For this review, take the finished solid that the model builds, in its own axes (mm). A direction names the side the tool comes from. Round coordinates to 2 decimals unless told otherwise and drop trailing zeros. Write each loop counter-clockwise with the first axis right and the second up, starting at its lowest first coordinate (ties: lowest second). Pieces come first, ordered by that corner, then holes. Notation, with made-up numbers: M 37.25,13.5 L 74.25,13.5 A9 cw 74.25,29.5 Z; hole C 22,0.25 d11. An arc over 180 degrees is marked long. Answer in a Markdown table with one row per item.
```python
from build123d import *

# Parameters (mm, degrees)
SKETCH1_W                      = 170
SKETCH1_H                      = 200
BOSS_EXTRUDE1_DEPTH            = 3
FILLET1_R                      = 3
F_3_0MM_DOWEL_HOLE1_AT_2_COUNT = 2
F_3_0MM_DOWEL_HOLE1_AT_2_PITCH = 15
F_3_0MM_DOWEL_HOLE1_AT_3_COUNT = 2
F_3_0MM_DOWEL_HOLE1_AT_3_PITCH = 75
F_3_0MM_DOWEL_HOLE1_AT_4_COUNT = 2
F_3_0MM_DOWEL_HOLE1_AT_4_PITCH = 90
F_3_0MM_DOWEL_HOLE1_AT_5_COUNT = 2
F_3_0MM_DOWEL_HOLE1_AT_5_PITCH = 60
F_3_0MM_DOWEL_HOLE1_AT_6_COUNT = 2
F_3_0MM_DOWEL_HOLE1_AT_6_PITCH = 75
FILLET1_OF_MIRROR1_R           = 3


with BuildPart() as part:
    # Sketch1 → Boss-Extrude1 (new body)
    with BuildSketch(Plane(origin=(0, 0, 0), x_dir=(1, 0, 0), z_dir=(0, 1, 0))):
        with Locations((-85, 0)):
            Rectangle(SKETCH1_W, SKETCH1_H)
        Polygon((-19.723082923, 85.294117647), (-19.723082923, 23.203626969), (-125.276917077, 85.294117647), align=None, mode=Mode.SUBTRACT)
        Polygon((-39.446165847, 11.601813484), (-145, 11.601813484), (-145, 73.692304163), align=None, mode=Mode.SUBTRACT)
        Polygon((-125.276917077, -85.294117647), (-19.723082923, -23.203626969), (-19.723082923, -85.294117647), align=None, mode=Mode.SUBTRACT)
        Polygon((-145, -11.601813484), (-39.446165847, -11.601813484), (-145, -73.692304163), align=None, mode=Mode.SUBTRACT)
    boss_extrude1 = extrude(amount=BOSS_EXTRUDE1_DEPTH)

    # Fillet1
    fillet1_edges = [part.edges().sort_by_distance(p)[0] for p in [
        (-19.723082923, 1.5, -23.203626969),
        (-19.723082923, 1.5, -85.294117647),
        (-125.276917077, 1.5, -85.294117647),
        (-39.446165847, 1.5, -11.601813484),
        (-145, 1.5, -73.692304163),
        (-145, 1.5, -11.601813484),
        (-39.446165847, 1.5, 11.601813484),
        (-145, 1.5, 11.601813484),
        (-145, 1.5, 73.692304163),
        (-19.723082923, 1.5, 23.203626969),
        (-125.276917077, 1.5, 85.294117647),
        (-19.723082923, 1.5, 85.294117647),
    ]]
    fillet(fillet1_edges, radius=FILLET1_R)

    # Sketch2 → Ø3.0mm Dowel Hole1 (revolve, cut)
    with BuildSketch(Plane(origin=(-156.575, 3, -7.5), x_dir=(0, 0, 1), z_dir=(1, 0, 0))):
        Polygon((0, 0), (0, 15.901290929), (1.5, 15), (1.5, 0), align=None)
    f_3_0mm_dowel_hole1 = revolve(axis=Axis((-156.575, 9.35, -7.5), (0, -1, 0)), mode=Mode.SUBTRACT)

    # Ø3.0mm Dowel Hole1 at 2: Ø3.0mm Dowel Hole1 ×2
    with Locations(*[(0, 0, i * F_3_0MM_DOWEL_HOLE1_AT_2_PITCH) for i in range(1, F_3_0MM_DOWEL_HOLE1_AT_2_COUNT)]):
        add(f_3_0mm_dowel_hole1, mode=Mode.SUBTRACT)

    # Ø3.0mm Dowel Hole1 at 3: Ø3.0mm Dowel Hole1 ×2
    with Locations(*[(0, 0, i * F_3_0MM_DOWEL_HOLE1_AT_3_PITCH) for i in range(1, F_3_0MM_DOWEL_HOLE1_AT_3_COUNT)]):
        add(f_3_0mm_dowel_hole1, mode=Mode.SUBTRACT)

    # Ø3.0mm Dowel Hole1 at 4: Ø3.0mm Dowel Hole1 ×2
    with Locations(*[(0, 0, i * F_3_0MM_DOWEL_HOLE1_AT_4_PITCH) for i in range(1, F_3_0MM_DOWEL_HOLE1_AT_4_COUNT)]):
        add(f_3_0mm_dowel_hole1, mode=Mode.SUBTRACT)

    # Ø3.0mm Dowel Hole1 at 5: Ø3.0mm Dowel Hole1 ×2
    with Locations(*[(0, 0, -i * F_3_0MM_DOWEL_HOLE1_AT_5_PITCH) for i in range(1, F_3_0MM_DOWEL_HOLE1_AT_5_COUNT)]):
        add(f_3_0mm_dowel_hole1, mode=Mode.SUBTRACT)

    # Ø3.0mm Dowel Hole1 at 6: Ø3.0mm Dowel Hole1 ×2
    with Locations(*[(0, 0, -i * F_3_0MM_DOWEL_HOLE1_AT_6_PITCH) for i in range(1, F_3_0MM_DOWEL_HOLE1_AT_6_COUNT)]):
        add(f_3_0mm_dowel_hole1, mode=Mode.SUBTRACT)

    # Mirror1: Boss-Extrude1, Ø3.0mm Dowel Hole1 across plane
    add(boss_extrude1.mirror(Plane(origin=(0, 0, 0), x_dir=(0, 0, 1), z_dir=(1, 0, 0))))
    add(f_3_0mm_dowel_hole1.mirror(Plane(origin=(0, 0, 0), x_dir=(0, 0, 1), z_dir=(1, 0, 0))), mode=Mode.SUBTRACT)

    # Mirror1 copy 1 sketch → Mirror1 copy 1 (revolve, cut)
    with BuildSketch(Plane(origin=(156.575, 3, 7.5), x_dir=(0, 0, 1), z_dir=(-1, 0, 0))):
        Polygon((0, 0), (0, -15.901290929), (1.5, -15), (1.5, 0), align=None)
    revolve(axis=Axis((156.575, 9.35, 7.5), (0, 1, 0)), mode=Mode.SUBTRACT)

    # Mirror1 copy 2 sketch → Mirror1 copy 2 (revolve, cut)
    with BuildSketch(Plane(origin=(156.575, 3, 67.5), x_dir=(0, 0, 1), z_dir=(-1, 0, 0))):
        Polygon((0, 0), (0, -15.901290929), (1.5, -15), (1.5, 0), align=None)
    revolve(axis=Axis((156.575, 9.35, 67.5), (0, 1, 0)), mode=Mode.SUBTRACT)

    # Mirror1 copy 3 sketch → Mirror1 copy 3 (revolve, cut)
    with BuildSketch(Plane(origin=(156.575, 3, 82.5), x_dir=(0, 0, 1), z_dir=(-1, 0, 0))):
        Polygon((0, 0), (0, -15.901290929), (1.5, -15), (1.5, 0), align=None)
    revolve(axis=Axis((156.575, 9.35, 82.5), (0, 1, 0)), mode=Mode.SUBTRACT)

    # Mirror1 copy 4 sketch → Mirror1 copy 4 (revolve, cut)
    with BuildSketch(Plane(origin=(156.575, 3, -67.5), x_dir=(0, 0, 1), z_dir=(-1, 0, 0))):
        Polygon((0, 0), (0, -15.901290929), (1.5, -15), (1.5, 0), align=None)
    revolve(axis=Axis((156.575, 9.35, -67.5), (0, 1, 0)), mode=Mode.SUBTRACT)

    # Mirror1 copy 5 sketch → Mirror1 copy 5 (revolve, cut)
    with BuildSketch(Plane(origin=(156.575, 3, -82.5), x_dir=(0, 0, 1), z_dir=(-1, 0, 0))):
        Polygon((0, 0), (0, -15.901290929), (1.5, -15), (1.5, 0), align=None)
    revolve(axis=Axis((156.575, 9.35, -82.5), (0, 1, 0)), mode=Mode.SUBTRACT)

    # Fillet1 of Mirror1
    fillet1_of_mirror1_edges = [part.edges().sort_by_distance(p)[0] for p in [
        (19.723082923, 1.5, -23.203626969),
        (19.723082923, 1.5, -85.294117647),
        (125.276917077, 1.5, -85.294117647),
        (39.446165847, 1.5, -11.601813484),
        (145, 1.5, -73.692304163),
        (145, 1.5, -11.601813484),
        (39.446165847, 1.5, 11.601813484),
        (145, 1.5, 11.601813484),
        (145, 1.5, 73.692304163),
        (19.723082923, 1.5, 23.203626969),
        (125.276917077, 1.5, 85.294117647),
        (19.723082923, 1.5, 85.294117647),
    ]]
    fillet(fillet1_of_mirror1_edges, radius=FILLET1_OF_MIRROR1_R)


solid = part.part
```
Q1. Mouldability with a two-part tool opening along Z and no side actions: class faces 3 (the face through (2, 3, -1)), 4 (the face through (95.351, 1.479, -44.487)) as +Z half, -Z half, draft (parallel to the pull), parting line (faces both ways), or undercut.
Found:
| item | result |
|---|---|
| face 3 | draft |
| face 4 | undercut |
Q2. Machinability: for faces 1 (the face through (2, 0, -1)), 2 (the face through (-94.07, 1.479, 43.733)), which of the approach directions +Z, -Z, +X, -X, +Y, -Y give a long, thin tool a straight path to every point of the face, cutting with its end or side? Answer none if there is none.
Found:
| item | result |
|---|---|
| face 1 | +Z, -Z, +X, -X, -Y |
| face 2 | +Y, -Y |
Q3. Take a section at C-C (y = 2.3). State how many separate pieces and enclosed holes the cut face has, then the cut area to 3 significant figures.
Found:
| item | result |
|---|---|
| separate pieces | 1 |
| enclosed holes | 20 |
| area | 41,900 mm² |
Q4. Take a section at A-A (z = 52). State the section outline as (x, y) points, then the cut area to 3 significant figures.
Found:
| item | result |
|---|---|
| outline | M -170,0 L -145,0 L -145,3 L -170,3 Z; M -108.12,0 L -68.68,0 L -68.68,3 L -108.12,3 Z; M -19.72,0 L 19.72,0 L 19.72,3 L -19.72,3 Z; M 68.68,0 L 108.12,0 L 108.12,3 L 68.68,3 Z; M 145,0 L 170,0 L 170,3 L 145,3 Z |
| area | 505 mm² |
Q5. Insertion check: P1, Ø4, axis at x = -156.575, z = 82.5, coming from the -Y side. The pin has a flat end and moves straight along its axis. Give the tip position at first contact, or say it passes through.
Found:
| item | result |
|---|---|
| P1 | y = 0 |
Q6. For probe 1 along X at (y, z) = (1.2, 82.5) (3 decimals); probe 2 along Z at (x, y) = (-82, 2.85); probe 3 along Z at (x, y) = (-26, 2.85), list the stretches that pass through material, from the lowest coordinate up.
Found:
| item | result |
|---|---|
| probe 1 | -170 to -158.075, -155.075 to -117.253, -19.73 to 19.73, 117.253 to 155.075, 158.075 to 170 |
| probe 2 | -100 to -85.29, -59.84 to -36.63, -11.6 to 11.6, 36.63 to 59.84, 85.29 to 100 |
| probe 3 | -100 to -85.29, -26.9 to 26.9, 85.29 to 100 |
Q7. Take a section at B-B (x = -87). State the section outline as (y, z) points, then the cut area to 3 significant figures.
Found:
| item | result |
|---|---|
| outline | M 0,-100 L 3,-100 L 3,-85.29 L 0,-85.29 Z; M 0,-62.78 L 3,-62.78 L 3,-39.57 L 0,-39.57 Z; M 0,-11.6 L 3,-11.6 L 3,11.6 L 0,11.6 Z; M 0,39.57 L 3,39.57 L 3,62.78 L 0,62.78 Z; M 0,85.29 L 3,85.29 L 3,100 L 0,100 Z |
| area | 297 mm² |
